```python
from build123d import *

# Parameters (mm, degrees)
SKETCH007_R          = 2.45
PAD005_DEPTH         = 1.6
PAD006_DEPTH         = 6
SKETCH058_W          = 3.1771358599
SKETCH058_H          = 6.2
POCKET021_DEPTH      = 1.6
POCKET021_DEPTH_BACK = 3


with BuildPart() as part:
    # Sketch007 → Pad005 (new body)
    with BuildSketch(Plane.YZ.offset(8.7)):
        with BuildLine():
            ThreePointArc((-6, 6), (-7.4371881489, -9.1), (-6, -24.2))
            Line((-6, -24.2), (0, -24.2))
            ThreePointArc((0, -24.2), (4.2426406871, -22.4426406871), (6, -18.2))
            Line((6, 0), (6, -18.2))
            ThreePointArc((6, 0), (4.2426406871, 4.2426406871), (0, 6))
            Line((-6, 6), (0, 6))
        make_face()
        Circle(SKETCH007_R, mode=Mode.SUBTRACT)
        with Locations((0, -18.2)):
            Circle(SKETCH007_R, mode=Mode.SUBTRACT)
    extrude(amount=-PAD005_DEPTH)

    # Sketch008 → Pad006 (join)
    with BuildSketch(Plane.YZ.offset(8.7)):
        with BuildLine():
            ThreePointArc((5.8114989668, -16.707860677), (3.6774423219, -13.4590699257), (0, -12.2))
            Line((-7.3771358599, -12.2), (0, -12.2))
            ThreePointArc((-7.3771358599, -6), (-7.4371881489, -9.1), (-7.3771358599, -12.2))
            Line((-7.3771358599, -6), (0, -6))
            ThreePointArc((0, -6), (3.6774423219, -4.7409300743), (5.8114989668, -1.492139323))
            Line((5.8114989668, -1.492139323), (6, -0.7579762707))
            Line((6, -0.7579762707), (6, -17.4420237293))
            Line((6, -17.4420237293), (5.8114989668, -16.707860677))
        make_face()
    extrude(amount=PAD006_DEPTH)

    # Sketch058 → Pocket021 (cut, two sides)
    with BuildSketch(Plane.YZ.offset(8.7)) as pocket021_sk:
        with BuildLine():
            Line((-2.6, 6), (-6, 6))
            ThreePointArc((-6, 6), (-6.167388681, 5.1009268767), (-6.3244944235, 4.2))
            Line((-2.6, 4.2), (-6.3244944235, 4.2))
            Line((-2.6, 6), (-2.6, 4.2))
        make_face()
        with BuildLine():
            Line((-6, -24.2), (-2.6, -24.2))
            Line((-2.6, -24.2), (-2.6, -22.4))
            Line((-2.6, -22.4), (-6.3244944235, -22.4))
            ThreePointArc((-6.3244944235, -22.4), (-6.167388681, -23.3009268767), (-6, -24.2))
        make_face()
        with Locations((-4.18856793, -9.1)):
            Rectangle(SKETCH058_W, SKETCH058_H)
    extrude(amount=-POCKET021_DEPTH, mode=Mode.SUBTRACT)
    extrude(pocket021_sk.sketch, amount=POCKET021_DEPTH_BACK, mode=Mode.SUBTRACT)


with BuildPart() as part_1:
    # Body006 placement: moved
    add(part.part.moved(Location((0, -72.6064407756, 0))))


solid = part_1.part
```
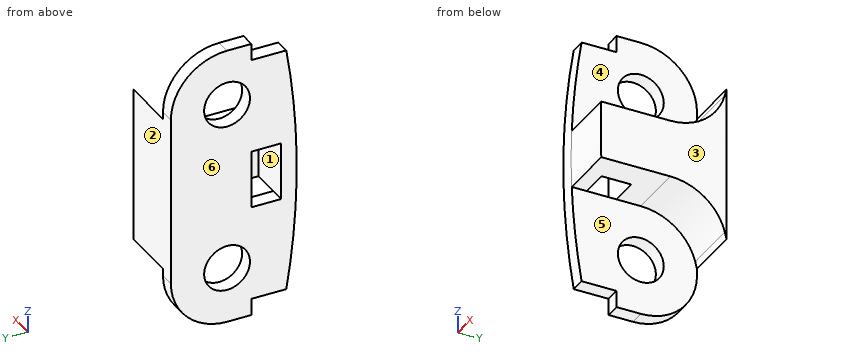
Check sheet for the modelled part. Datum: model origin and axes. Units: mm. Face numbers are marked on the shaded views. A direction names the side the tool comes from. Coordinates: 2 decimals unless noted, no trailing zeros. Order: outer loops, then holes, each group sorted by start corner. A loop starts at its lowest first (then second) coordinate and runs counter-clockwise, first axis right, second up. Notation, with made-up numbers: M 42.25,-28 L 50.25,-28 A32 ccw 50.25,10 Z; hole C 10.5,59 d11. An arc over 180 degrees is marked long. Write each question's results on one line, items separated by ' | '. Start each with the question number.
1. Mould release check, pull along Y, two halves, no side actions. Record for the marked faces 1, 2 and 3: +Y half, -Y half, draft (parallel to the pull), parting line (faces both ways), or undercut.
2. Access from +Z, -Z, +X, -X, +Y, -Y to the whole of each face (thin tool, end or side, straight path). Record for the marked faces 4, 5 and 6.
3. Material ranges on probe 1 along X at (y, z) = (-77, -21); probe 2 along Z at (x, y) = (13.25, -74.75); probe 3 along X at (y, z) = (-75.75, -11.5), recorded low to high.
4. Go/stop test with flat-tipped pins: P1, Ø1.3, axis at x = 8, y = -76.5, coming from the +Z side; P2, Ø1.8, axis at x = 8, y = -77, coming from the -Z side; P3, Ø1.8, axis at x = 11.5, y = -75, coming from the -Z side. Record where each tip stops, or that it passes through.
5. Cross-section at C-C on x = 13.5. Record the cut outline in (y, z), and give its area (3 significant figures).
6. Cross-section at A-A on y = -77.5. Record the cut outline in (x, z).
7. Cross-section at B-B on x = 8. Record the cut outline in (y, z), and give its area (3 significant figures).
8. Cross-section at D-D on z = -19.5. Record the cut outline in (x, y).
Checks:
1) face 1: undercut | face 2: +Y half | face 3: draft
2) face 4: +Z, +X, -Y | face 5: -Z, +X, -Y | face 6: +Z, -Z, -X, +Y, -Y
3) probe 1: x = 7.1 to 8.7 | probe 2: z = -12.2 to -6 | probe 3: x = 11.7 to 14.7
4) P1: stops at z = 4.2 | P2: stops at z = -22.4 | P3: stops at z = -12.2
5) outline: M -79.98,-12.2 L -72.61,-12.2 A6 cw -66.79,-16.71 L -66.61,-17.44 L -66.61,-0.76 L -66.79,-1.49 A6 cw -72.61,-6 L -79.98,-6 A80.04 ccw Z | area: 98.6 mm²
6) outline: M 7.1,-22.4 L 8.7,-22.4 L 8.7,-12.2 L 7.1,-12.2 Z; M 7.1,-6 L 8.7,-6 L 8.7,4.2 L 7.1,4.2 Z; M 11.7,-12.2 L 14.7,-12.2 L 14.7,-6 L 11.7,-6 Z
7) outline: M -78.93,-22.4 L -75.21,-22.4 L -75.21,-24.2 L -72.61,-24.2 A6 ccw -66.61,-18.2 L -66.61,0 A6 ccw -72.61,6 L -75.21,6 L -75.21,4.2 L -78.93,4.2 A80.04 ccw Z; hole M -78.38,-12.2 L -75.21,-12.2 L -75.21,-6 L -78.38,-6 Z; hole C -72.61,-18.2 d4.9; hole C -72.61,0 d4.9 | area: 306 mm²
8) outline: M 7.1,-79.37 L 8.7,-79.37 L 8.7,-74.68 L 7.1,-74.68 Z; M 7.1,-70.53 L 8.7,-70.53 L 8.7,-66.75 L 7.1,-66.75 Z
